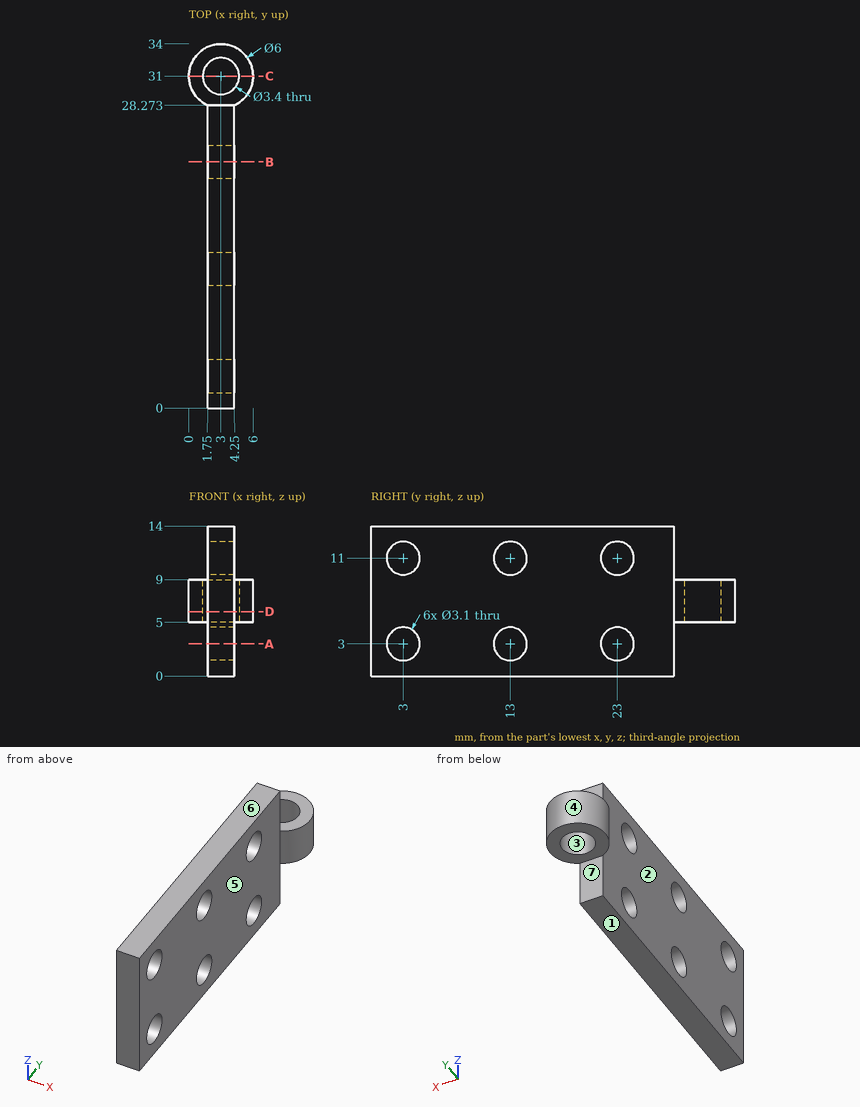
Input: dimensioned drawing with shaded views. Units: mm. Origin: part minimum x, y, z. A direction names the side the tool comes from. Round coordinates to 2 decimals unless told otherwise and drop trailing zeros. Loops run counter-clockwise (first coordinate to the right, second up) from the corner with the lowest first, then second, coordinate; pieces in that order, holes last. Notation, with made-up numbers: M 52.25,2 L 101.25,2 A24 ccw 101.25,25 Z; hole C 81.5,33 d1. An arc over 180 degrees is marked long. Return JSON: item names as keys, results as strings. Group by question number.
1. Reachability of the marked faces 5, 6 and 7 from +Z, -Z, +X, -X, +Y, -Y: full face, straight path, thin tool, end or side. Return the list, or none.
2. Section query B-B on y = 23. Output: boundary loops of the cut face in (x, z).
3. Material intervals for line 1 along Y through (x, z) = (2.75, 11); line 2 along Z through (x, y) = (3, 13); line 3 along Z through (x, y) = (2.1, 14) (1 decimal), sorted ascending. Write a range as from..to.
4. Section query D-D on z = 6. Output: boundary loops of the cut face in (x, y), and give its area (3 significant figures).
5. Section query C-C on y = 31. Output: boundary loops of the cut face in (x, z).
6. Section query A-A on z = 3. Output: boundary loops of the cut face in (x, y).
7. Mould query, pull axis X, two halves, no side actions, for the marked faces 1, 2, 3 and 4. Classes: released by +X, released by -X, zero draft, split by the parting line, or undercut.
8. Pin query (flat end, axial travel): pin 1 (1.2 mm diameter, centred on x = 3, z = 2, fed in from +Y); pin 2 (3 mm diameter, centred on x = 4.5, y = 31.5, fed in from -Z); pin 3 (4 mm diameter, centred on y = 13, z = 11, fed in from +X). Return the tip coordinate at first contact, or that it passes through.
Checks:
{
 "1": {"face 5": "+Z, -Z, +X, -Y", "face 6": "+Z, +X, -X, +Y, -Y", "face 7": "-Z, +X, -X, +Y"},
 "2": {"outline": "M 1.75,0 L 4.25,0 L 4.25,1.45 L 1.75,1.45 Z; M 1.75,4.55 L 4.25,4.55 L 4.25,9.45 L 1.75,9.45 Z; M 1.75,12.55 L 4.25,12.55 L 4.25,14 L 1.75,14 Z"},
 "3": {"line 1": "y = 0..1.45, 4.55..11.45, 14.55..21.45, 24.55..28.27", "line 2": "z = 0..1.45, 4.55..9.45, 12.55..14", "line 3": "z = 0..1.8, 4.2..9.8, 12.2..14"},
 "4": {"outline": "M 1.75,0 L 4.25,0 L 4.25,28.27 A3 ccw long 1.75,28.27 Z; hole C 3,31 d3.4", "area": "89.4 mm²"},
 "5": {"outline": "M 0,5 L 1.3,5 L 1.3,9 L 0,9 Z; M 4.7,5 L 6,5 L 6,9 L 4.7,9 Z"},
 "6": {"outline": "M 1.75,0 L 4.25,0 L 4.25,1.45 L 1.75,1.45 Z; M 1.75,4.55 L 4.25,4.55 L 4.25,11.45 L 1.75,11.45 Z; M 1.75,14.55 L 4.25,14.55 L 4.25,21.45 L 1.75,21.45 Z; M 1.75,24.55 L 4.25,24.55 L 4.25,28.27 L 1.75,28.27 Z"},
 "7": {"face 1": "zero draft", "face 2": "released by -X", "face 3": "undercut", "face 4": "split by the parting line"},
 "8": {"pin 1": "stops at y = 28.27", "pin 2": "stops at z = 5", "pin 3": "stops at x = 4.25"}
}
